Verification items for the finished model (mm, model axes). Face numbers are marked on the shaded views. A direction names the side the tool comes from. Round coordinates to 2 decimals unless told otherwise and drop trailing zeros. Write each loop counter-clockwise with the first axis right and the second up, starting at its lowest first coordinate (ties: lowest second). Pieces come first, ordered by that corner, then holes. Notation, with made-up numbers: (-34.5, 8) - (7.5, 8) arc R14 ccw to (7.5, 29) - close; hole circle Ø3 at (-2.75, 44.5). An arc over 180 degrees is marked (long way). Write each question's results on one line, items separated by ' | '.
```python
from build123d import *

# Parameters (mm, degrees)
CYLINDER_R        = 1
CYLINDER_DEPTH    = 28
CYLINDER004_R     = 2
CYLINDER004_DEPTH = 10
CYLINDER005_R     = 2
CYLINDER005_DEPTH = 10
CYLINDER003_R     = 2
CYLINDER003_DEPTH = 10
CYLINDER001_R     = 1
CYLINDER001_DEPTH = 28
CYLINDER002_R     = 2
CYLINDER002_DEPTH = 10
BOX002_W          = 16
BOX002_H          = 23
BOX002_DEPTH      = 12.5
BOX001_W          = 10
BOX001_H          = 35
BOX001_DEPTH      = 12.5
BOX_W             = 24
BOX_H             = 50
BOX_DEPTH         = 3
FILLET_R          = 2
FILLET001_R       = 1
FILLET002_R       = 2
FILLET003_R       = 2


with BuildPart() as cylinder:
    # Cylinder → Cylinder (new body)
    with BuildSketch(Plane(origin=(0, 11.25, 9.25), x_dir=(0, 0, -1), z_dir=(1, 0, 0))):
        Circle(CYLINDER_R)
    extrude(amount=CYLINDER_DEPTH)


with BuildPart() as cylinder004:
    # Cylinder004 → Cylinder004 (new body)
    with BuildSketch(Plane(origin=(20, 4, 0), x_dir=(1, 0, 0), z_dir=(0, 0, 1))):
        Circle(CYLINDER004_R)
    extrude(amount=CYLINDER004_DEPTH)


with BuildPart() as cylinder005:
    # Cylinder005 → Cylinder005 (new body)
    with BuildSketch(Plane(origin=(20, 46, 0), x_dir=(1, 0, 0), z_dir=(0, 0, 1))):
        Circle(CYLINDER005_R)
    extrude(amount=CYLINDER005_DEPTH)


with BuildPart() as cylinder003:
    # Cylinder003 → Cylinder003 (new body)
    with BuildSketch(Plane(origin=(4, 46, 0), x_dir=(1, 0, 0), z_dir=(0, 0, 1))):
        Circle(CYLINDER003_R)
    extrude(amount=CYLINDER003_DEPTH)


with BuildPart() as cylinder001:
    # Cylinder001 → Cylinder001 (new body)
    with BuildSketch(Plane(origin=(0, 38.75, 9.25), x_dir=(0, 0, -1), z_dir=(1, 0, 0))):
        Circle(CYLINDER001_R)
    extrude(amount=CYLINDER001_DEPTH)


with BuildPart() as fusion001:
    # Cylinder002 → Cylinder002 (new body)
    with BuildSketch(Plane(origin=(4, 4, 0), x_dir=(1, 0, 0), z_dir=(0, 0, 1))):
        Circle(CYLINDER002_R)
    extrude(amount=CYLINDER002_DEPTH)

    # Fusion001: union Cylinder, Cylinder004, Cylinder005, Cylinder003, Cylinder001
    add(cylinder.part)
    add(cylinder004.part)
    add(cylinder005.part)
    add(cylinder003.part)
    add(cylinder001.part)


with BuildPart() as cube001:
    # Box002 → Box002 (new body)
    with BuildSketch(Plane(origin=(7, 13.5, 3), x_dir=(1, 0, 0), z_dir=(0, 0, 1))):
        with Locations((8, 11.5)):
            Rectangle(BOX002_W, BOX002_H)
    extrude(amount=BOX002_DEPTH)


with BuildPart() as cut:
    # Box001 → Box001 (new body)
    with BuildSketch(Plane(origin=(7, 7.5, 3), x_dir=(1, 0, 0), z_dir=(0, 0, 1))):
        with Locations((5, 17.5)):
            Rectangle(BOX001_W, BOX001_H)
    extrude(amount=BOX001_DEPTH)

    # Cut: cut Cube001
    add(cube001.part, mode=Mode.SUBTRACT)


with BuildPart() as fillet003:
    # Box → Box (new body)
    with BuildSketch(Plane.XY):
        with Locations((12, 25)):
            Rectangle(BOX_W, BOX_H)
    extrude(amount=BOX_DEPTH)

    # Fillet
    fillet_edges = [fillet003.edges().sort_by_distance(p)[0] for p in [
        (0, 0, 1.5),
        (0, 50, 1.5),
        (24, 0, 1.5),
        (24, 50, 1.5),
    ]]
    fillet(fillet_edges, radius=FILLET_R)

    # Fusion: union Cut
    add(cut.part)

    # Cut001: cut Fusion001
    add(fusion001.part, mode=Mode.SUBTRACT)

    # Fillet001
    fillet001_edges = [fillet003.edges().sort_by_distance(p)[0] for p in [
        (12, 13.5, 3),
        (12, 36.5, 3),
    ]]
    fillet(fillet001_edges, radius=FILLET001_R)

    # Fillet002
    fillet002_edges = [fillet003.edges().sort_by_distance(p)[0] for p in [
        (12, 7.5, 3),
        (12, 42.5, 3),
    ]]
    fillet(fillet002_edges, radius=FILLET002_R)

    # Fillet003
    fillet003_edges = [fillet003.edges().sort_by_distance(p)[0] for p in [
        (12, 7.5, 15.5),
        (12, 42.5, 15.5),
    ]]
    fillet(fillet003_edges, radius=FILLET003_R)


solid = fillet003.part
```
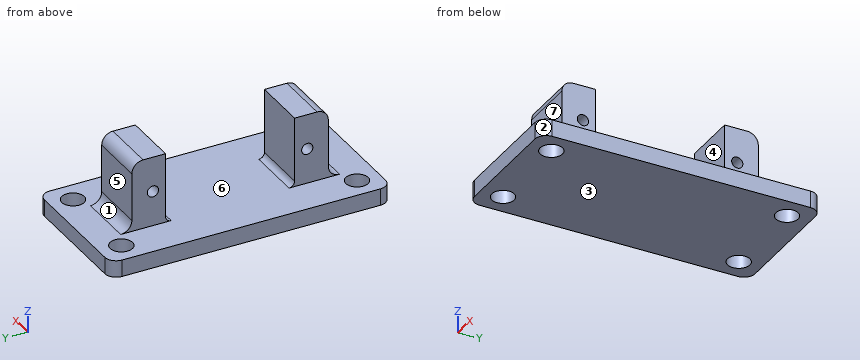
(1) Go/stop test with flat-tipped pins: pin 1 Ø7 at (x, z) = (12, 8) entering from +Y; pin 2 Ø5 at (x, y) = (4, 4) entering from +Z; pin 3 Ø1 at (y, z) = (10.5, 9.5) entering from +X; pin 4 Ø8 at (y, z) = (29.5, 4) entering from -X. Record where each tip stops, or that it passes through.
Answer:
pin 1: y = 42.56 | pin 2: z = 3 | pin 3: x = 17 | pin 4: x = 0
(2) Thickness scan on L1, parallel to Y at x = 11.75, z = 9.25; L2, parallel to X at y = 4, z = 1; L3, parallel to Y at x = 4, z = 2.05. Record the ranges inside material, lowest first.
Answer:
L1: 7.5 to 10.25, 12.25 to 13.5, 36.5 to 37.75, 39.75 to 42.5 | L2: 0 to 2, 6 to 18, 22 to 24 | L3: 0 to 2, 6 to 44, 48 to 50
(3) Section check B-B (z = 7.25). Record the cut outline in (x, y), plus the area to 3 significant figures.
Answer:
outline: (7, 7.5) - (17, 7.5) - (17, 13.5) - (7, 13.5) - close; (7, 36.5) - (17, 36.5) - (17, 42.5) - (7, 42.5) - close | area: 120 mm2
(4) Mould release check, pull along Y, two halves, no side actions. Record for the marked faces 1, 2, 3 and 4: released by +Y, released by -Y, zero draft, split by the parting line, or undercut.
Answer:
face 1: released by +Y | face 2: released by -Y | face 3: zero draft | face 4: undercut
(5) Section check A-A (y = 46). Record the cut outline in (x, z), plus the area to 3 significant figures.
Answer:
outline: (0, 0) - (2, 0) - (2, 3) - (0, 3) - close; (6, 0) - (18, 0) - (18, 3) - (6, 3) - close; (22, 0) - (24, 0) - (24, 3) - (22, 3) - close | area: 48.0 mm2
(6) Section check C-C (x = 4). Record the cut outline in (y, z).
Answer:
outline: (0, 0) - (2, 0) - (2, 3) - (0, 3) - close; (6, 0) - (44, 0) - (44, 3) - (6, 3) - close; (48, 0) - (50, 0) - (50, 3) - (48, 3) - close
(7) Section check D-D (y = 11.25). Record the cut outline in (x, z), plus the area to 3 significant figures.
Answer:
outline: (0, 0) - (24, 0) - (24, 3) - (17, 3) - (17, 8.25) - (7, 8.25) - (7, 3) - (0, 3) - close; (7, 10.25) - (17, 10.25) - (17, 15.5) - (7, 15.5) - close | area: 177 mm2
(8) Set-up check for the marked faces 5, 6 and 7: record each of +Z, -Z, +X, -X, +Y, -Y from which the full face is reachable in a straight line by a thin tool's end or side.
Answer:
face 5: +Z, +X, -X, +Y | face 6: +Z | face 7: +Z, +X, -X, -Y
